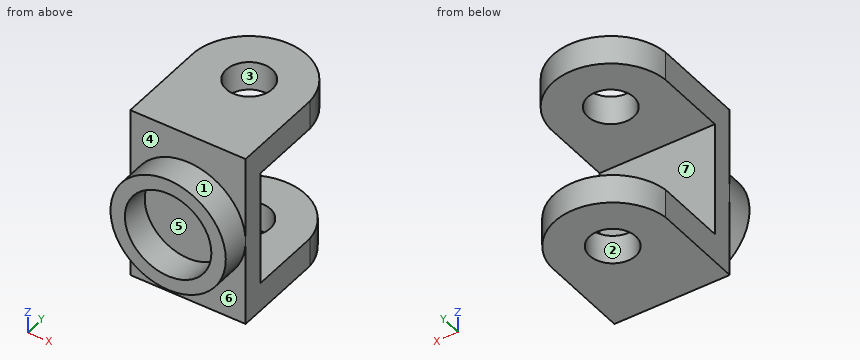
```python
from build123d import *

# Parameters (mm, degrees)
SKETCH_W      = 80
SKETCH_H      = 120
PAD_DEPTH     = 7.5
SKETCH001_R   = 16
PAD001_DEPTH  = 20
SKETCH002_R   = 16
PAD002_DEPTH  = 20
SKETCH003_R   = 40
SKETCH003_R_2 = 30
PAD003_DEPTH  = 20


with BuildPart() as part:
    # Sketch → Pad (new body, symmetric)
    with BuildSketch(Plane.XZ):
        with Locations((-1.950326, 25.453721)):
            Rectangle(SKETCH_W, SKETCH_H)
    extrude(amount=PAD_DEPTH, both=True)

    # Sketch001 (on Face3 of Pad) → Pad001 (join)
    with BuildSketch(Plane(origin=(0, 0, -34.546279), x_dir=(1, 0, 0), z_dir=(0, 0, -1))):
        with BuildLine():
            Line((-41.950326, -7.5), (38.049674, -7.5))
            Line((38.049674, -7.5), (38.049674, -57.5))
            ThreePointArc((-41.950326, -57.5), (-1.950326, -92.751304), (38.049674, -57.5))
            Line((-41.950326, -7.5), (-41.950326, -57.5))
        make_face()
        with Locations((-1.950326, -52.431456)):
            Circle(SKETCH001_R, mode=Mode.SUBTRACT)
    extrude(amount=-PAD001_DEPTH)

    # Sketch002 (on Face1 of Pad001) → Pad002 (join)
    with BuildSketch(Plane(origin=(0, 0, 85.453721), x_dir=(-1, 0, 0), z_dir=(0, 0, 1))):
        with BuildLine():
            Line((-38.049674, -57.5), (-38.049674, -7.5))
            Line((-38.049674, -7.5), (41.950326, -7.5))
            Line((41.950326, -7.5), (41.950326, -57.5))
            ThreePointArc((-38.049674, -57.5), (1.950326, -94.541734), (41.950326, -57.5))
        make_face()
        with Locations((1.950326, -54.423606)):
            Circle(SKETCH002_R, mode=Mode.SUBTRACT)
    extrude(amount=-PAD002_DEPTH)

    # Sketch003 (on Face5 of Pad002) → Pad003 (join)
    with BuildSketch(Plane.XZ.offset(7.5)):
        with Locations((-1.950326, 25.453721)):
            Circle(SKETCH003_R)
        with Locations((-1.950326, 25.453721)):
            Circle(SKETCH003_R_2, mode=Mode.SUBTRACT)
    extrude(amount=PAD003_DEPTH)


solid = part.part
```
Here's how the part is built. I have some questions about the finished solid (model axes, mm). Face numbers are marked on the shaded views. A direction names the side the tool comes from. Round coordinates to 2 decimals unless told otherwise and drop trailing zeros. Write each loop counter-clockwise with the first axis right and the second up, starting at its lowest first coordinate (ties: lowest second). Pieces come first, ordered by that corner, then holes. Notation, with made-up numbers: M 83,20 L 99,20 A23 ccw 99,59 Z; hole C 62.5,14 d7. An arc over 180 degrees is marked long. Answer as CSV lines item,"result". Start each with the question number.
1. I'm going to push flat-ended pins straight in: pin 1 Ø5 at (x, z) = (-29, 66.5) entering from +Y; pin 2 Ø8 at (x, z) = (21, 8.5) entering from +Y; pin 3 Ø6 at (x, z) = (-11.5, -19.5) entering from +Y. Where does each tip first touch, or does it pass through?
2. Suppose I cut it at A-A on y = 34. Write out the boundary of the cut face in (x, z), then the cut area to 3 significant figures.
3. On a 3-axis mill with a long thin cutter (end or side, diameter ignored), from which of +Z, -Z, +X, -X, +Y, -Y can I reach the whole of each face in a straight line? I mean the marked faces 5, 6 and 7. Say none if no direction works.
4. Suppose I cut it at D-D on z = 62.5. Write out the boundary of the cut face in (x, y), then the cut area to 3 significant figures.
5. Thinking about a two-plate mould opening in Y: for the marked faces 1, 2, 3 and 4, which applies, released by +Y, released by -Y, zero draft, split by the parting line, or undercut?
6. Suppose I cut it at C-C on z = 75. Write out the boundary of the cut face in (x, y), then the cut area to 3 significant figures.
7. Suppose I cut it at B-B on x = -4.5. Write out the boundary of the cut face in (y, z), then the cut area to 3 significant figures.
8. I need wall thicknesses on probe 1 along Z at (x, y) = (34.5, 39); probe 2 along Y at (x, z) = (-15.5, 8.5); probe 3 along Y at (x, z) = (26.5, 14). Which ranges of each line are inside material? Lowest first, please.
Check result:
1,pin 1,"stops at y = 86.15"
1,pin 2,"stops at y = 7.5"
1,pin 3,"stops at y = 92.22"
2,outline,"M -41.95,-34.55 L 38.05,-34.55 L 38.05,-14.55 L -41.95,-14.55 Z; M -41.95,65.45 L 38.05,65.45 L 38.05,85.45 L -41.95,85.45 Z"
2,area,"3,200 mm2"
3,face 5,"-Y"
3,face 6,"-Z, -Y"
3,face 7,"+X, -X, +Y"
4,outline,"M -41.95,-7.5 L -17.04,-7.5 L -17.04,-27.5 L 13.14,-27.5 L 13.14,-7.5 L 38.05,-7.5 L 38.05,7.5 L -41.95,7.5 Z"
4,area,"1,800 mm2"
5,face 1,"zero draft"
5,face 2,"undercut"
5,face 3,"undercut"
5,face 4,"released by -Y"
6,outline,"M -41.95,-7.5 L 38.05,-7.5 L 38.05,57.5 A40.12 ccw -41.95,57.5 Z; hole C -1.95,54.42 d32"
6,area,"6,680 mm2"
7,outline,"M -27.5,-14.46 L -7.5,-14.46 L -7.5,-34.55 L 36.64,-34.55 L 36.64,-14.55 L 7.5,-14.55 L 7.5,65.45 L 38.63,65.45 L 38.63,85.45 L -7.5,85.45 L -7.5,65.37 L -27.5,65.37 L -27.5,55.35 L -7.5,55.35 L -7.5,-4.44 L -27.5,-4.44 Z; M 68.23,-34.55 L 92.67,-34.55 L 92.67,-14.55 L 68.23,-14.55 Z; M 70.22,65.45 L 94.46,65.45 L 94.46,85.45 L 70.22,85.45 Z"
7,area,"4,380 mm2"
8,probe 1,"z = -34.55 to -14.55, 65.45 to 85.45"
8,probe 2,"y = -7.5 to 7.5"
8,probe 3,"y = -27.5 to 7.5"
